Source: three-view drawing plus pictorial views. Frame: mm from the lowest corner of the part. A direction names the side the tool comes from. Coordinates: 2 decimals unless noted, no trailing zeros. Order: outer loops, then holes, each group sorted by start corner. A loop starts at its lowest first (then second) coordinate and runs counter-clockwise, first axis right, second up. Notation, with made-up numbers: (-24.5, -27) - (-11.5, -27) arc R19 cw to (-11.5, -2) - close; hole circle Ø10 at (86, -37). An arc over 180 degrees is marked (long way). One line per question, with ' | ' between items.
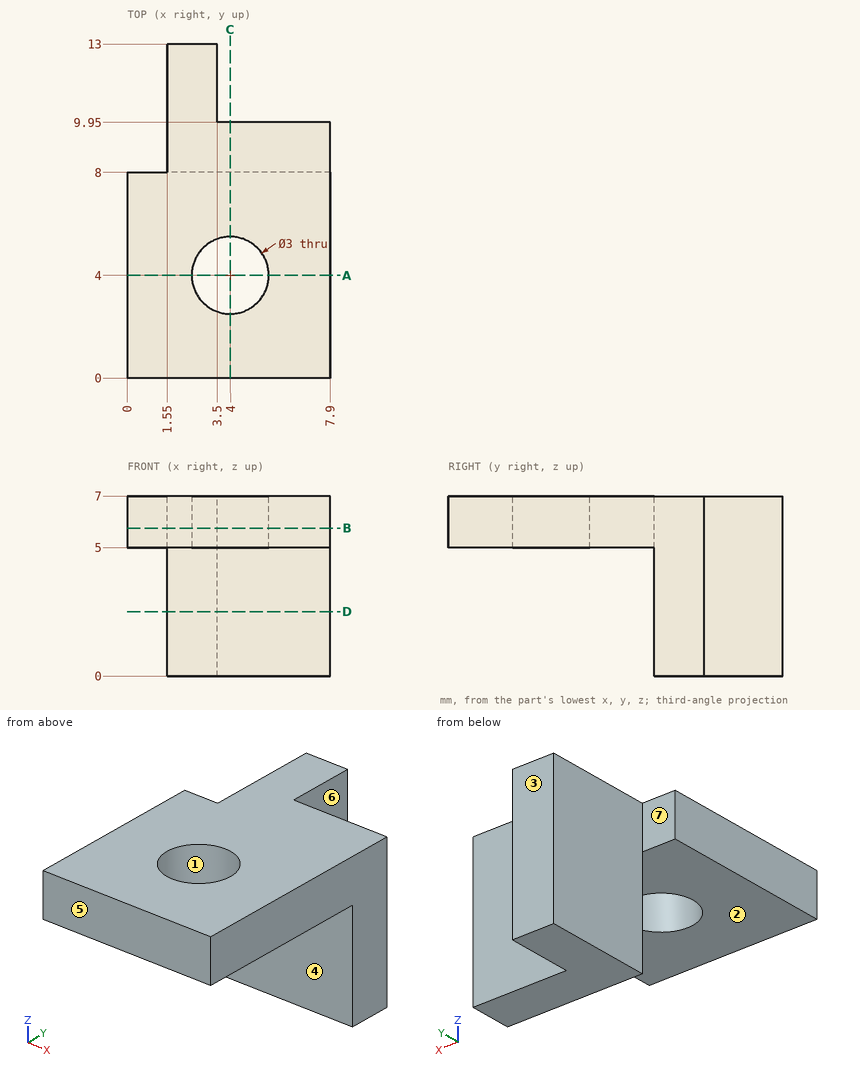
(1) Cut plane D-D (z = 2.5). Return the cut outline in (x, y).
Taken from the geometry:
outline: (1.55, 8) - (7.9, 8) - (7.9, 9.95) - (3.5, 9.95) - (3.5, 13) - (1.55, 13) - close
(2) Material intervals for L1, parallel to Y at x = 4, z = 5.7; L2, parallel to X at y = 4, z = 5.6; L3, parallel to Y at x = 2.5, z = 4.5, sorted ascending. Write a range as from..to.
Taken from the geometry:
L1: y = 0..2.5, 5.5..9.95 | L2: x = 0..2.5, 5.5..7.9 | L3: y = 8..13
(3) Pin query (flat end, axial travel): P1, Ø1.5, axis at y = 12, z = 2.5, coming from the +X side; P2, Ø2.5, axis at y = 11.5, z = 4.5, coming from the -X side; P3, Ø1.3, axis at x = 5, z = 3.5, coming from the +Y side. Return the tip coordinate at first contact, or that it passes through.
Taken from the geometry:
P1: stops at x = 3.5 | P2: stops at x = 1.55 | P3: stops at y = 9.95
(4) Set-up query: the marked faces 4, 5, 6 and 7. Return all of +Z, -Z, +X, -X, +Y, -Y with unobstructed straight access to the full face (end or side cutting, diameter ignored); none if empty.
Taken from the geometry:
face 4: -Z, +X, -X, -Y | face 5: +Z, -Z, +X, -X, -Y | face 6: +Z, -Z, +X, +Y | face 7: +Z, -Z, -X, +Y
(5) Cut plane B-B (z = 5.75). Return the cut outline in (x, y).
Taken from the geometry:
outline: (0, 0) - (7.9, 0) - (7.9, 9.95) - (3.5, 9.95) - (3.5, 13) - (1.55, 13) - (1.55, 8) - (0, 8) - close; hole circle Ø3 at (4, 4)
(6) Pull-direction query (Y, two-part tool) for the marked faces 1, 2 and 3; classes: pulls with the +Y half, pulls with the -Y half, needs draft (parallel to the pull), parting line crosses it, or undercut.
Taken from the geometry:
face 1: undercut | face 2: needs draft | face 3: pulls with the +Y half
(7) Cut plane A-A (y = 4). Return the cut outline in (x, z), and give its area (3 significant figures).
Taken from the geometry:
outline: (0, 5) - (2.5, 5) - (2.5, 7) - (0, 7) - close; (5.5, 5) - (7.9, 5) - (7.9, 7) - (5.5, 7) - close | area: 9.80 mm²
(8) Cut plane C-C (x = 4). Return the cut outline in (y, z), and give its area (4 significant figures).
Taken from the geometry:
outline: (0, 5) - (2.5, 5) - (2.5, 7) - (0, 7) - close; (5.5, 5) - (8, 5) - (8, 0) - (9.95, 0) - (9.95, 7) - (5.5, 7) - close | area: 23.65 mm²
